Can you work these out from the drawing? Everything is in mm from the part's minimum corner. A direction names the side the tool comes from. Coordinates: 2 decimals unless noted, no trailing zeros. Loops run counter-clockwise (first coordinate to the right, second up) from the corner with the lowest first, then second, coordinate; pieces in that order, holes last. Notation, with made-up numbers: (13.5, -5) - (48.5, -5) arc R23 cw to (48.5, 32) - close; hole circle Ø6 at (36.25, 18.5). An arc over 180 degrees is marked (long way). Put each result on its own line as item: value. Start each with the question number.
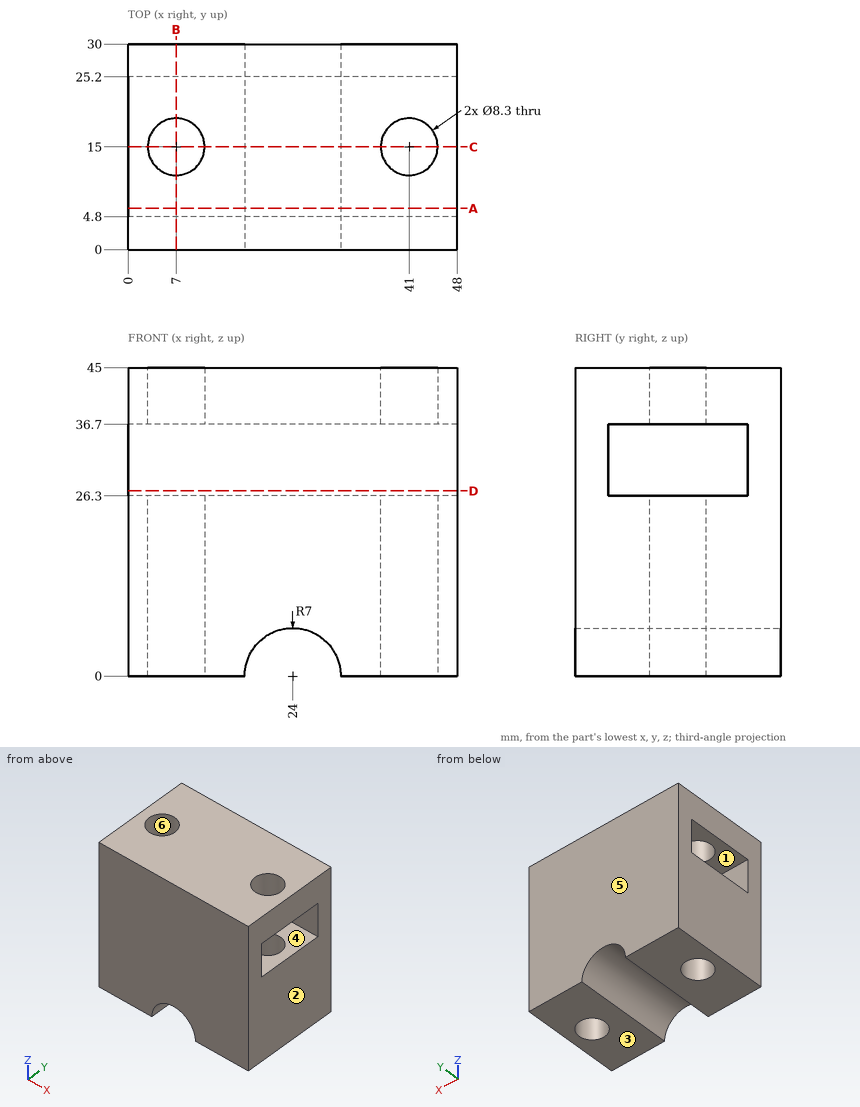
(1) Which directions (+Z, -Z, +X, -X, +Y, -Y) give clear straight access to the entire face, cutting with the end or side of a thin tool? Please do the marked faces 1 and 2.
(2) I want a section at B-B on x = 7. List the corners of the cut face in (y, z) for me, and give its area (3 significant figures).
(3) If we mould it in two halves opening along Y, with no side actions, what happens to the marked faces 3, 4, 5 and 6? For each: pulls with the +Y half, pulls with the -Y half, needs draft (parallel to the pull), parting line crosses it, or undercut.
(4) I want a section at C-C on y = 15. List the corners of the cut face in (x, z) for me, and give its area (3 significant figures).
(5) I want a section at D-D on z = 27. List the corners of the cut face in (x, y) for me, and give its area (3 significant figures).
(6) I want a section at A-A on y = 6. List the corners of the cut face in (x, z) for me.
(7) I need wall thicknesses on L1, parallel to Y at x = 33, z = 35; L2, parallel to X at y = 17.5, z = 20; L3, parallel to X at y = 13, z = 12.5. Which ranges of each line are inside material? Lowest first, please. Write a range as [from, to].
Answer sheet:
1. face 1: +X, -X
1. face 2: +Z, -Z, +X, +Y, -Y
2. outline: (0, 0) - (10.85, 0) - (10.85, 26.3) - (4.8, 26.3) - (4.8, 36.7) - (10.85, 36.7) - (10.85, 45) - (0, 45) - close; (19.15, 0) - (30, 0) - (30, 45) - (19.15, 45) - (19.15, 36.7) - (25.2, 36.7) - (25.2, 26.3) - (19.15, 26.3) - close
2. area: 851 mm^2
3. face 3: needs draft
3. face 4: undercut
3. face 5: pulls with the +Y half
3. face 6: undercut
4. outline: (0, 0) - (2.85, 0) - (2.85, 26.3) - (0, 26.3) - close; (0, 36.7) - (2.85, 36.7) - (2.85, 45) - (0, 45) - close; (11.15, 0) - (17, 0) arc R7 cw to (31, 0) - (36.85, 0) - (36.85, 26.3) - (11.15, 26.3) - close; (11.15, 36.7) - (36.85, 36.7) - (36.85, 45) - (11.15, 45) - close; (45.15, 0) - (48, 0) - (48, 26.3) - (45.15, 26.3) - close; (45.15, 36.7) - (48, 36.7) - (48, 45) - (45.15, 45) - close
4. area: 1,010 mm^2
5. outline: (0, 0) - (48, 0) - (48, 4.8) - (0, 4.8) - close; (0, 25.2) - (48, 25.2) - (48, 30) - (0, 30) - close
5. area: 461 mm^2
6. outline: (0, 0) - (17, 0) arc R7 cw to (31, 0) - (48, 0) - (48, 26.3) - (0, 26.3) - close; (0, 36.7) - (48, 36.7) - (48, 45) - (0, 45) - close
7. L1: y = [0, 4.8], [25.2, 30]
7. L2: x = [0, 3.69], [10.31, 37.69], [44.31, 48]
7. L3: x = [0, 3.36], [10.64, 37.36], [44.64, 48]
